Part model, mm, in its own coordinate system. Face numbers are marked on the shaded views. A direction names the side the tool comes from. Round coordinates to 2 decimals unless told otherwise and drop trailing zeros. Loops run counter-clockwise (first coordinate to the right, second up) from the corner with the lowest first, then second, coordinate; pieces in that order, holes last.
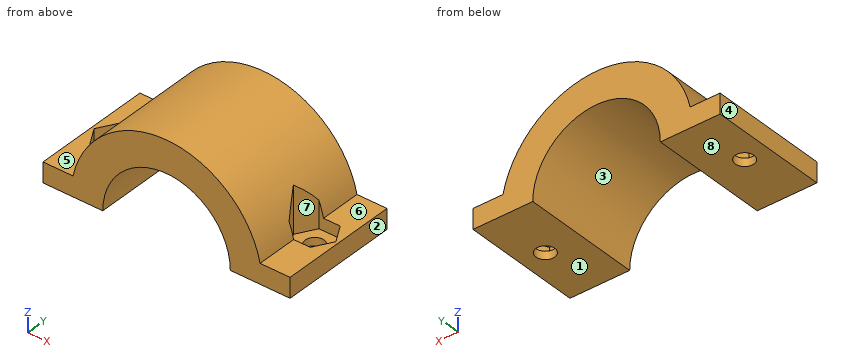
from build123d import *

# Parameters (mm, degrees)
BOSS_EXTRUDE1_DEPTH   = 30
CUT_EXTRUDE1_DEPTH    = 50
SKETCH2_7_R           = 2.35
CUT_EXTRUDE5_DEPTH    = 5
SKETCH2_10_R          = 2.35
CUT_EXTRUDE8_DEPTH    = 3
BODY_MOVE_COPY1_ANGLE = 90


with BuildPart() as part:
    # Sketch1 → Boss-Extrude1 (new body)
    with BuildSketch(Plane(origin=(0, 0, 0), x_dir=(1, 0, 0), z_dir=(0, 1, 0))):
        with BuildLine():
            Line((0, -16), (0, -31))
            Line((0, -31), (-5, -31))
            Line((-5, -31), (-5, -23.473389189))
            ThreePointArc((-5, -23.473389189), (-24, 0), (-5, 23.473389189))
            Line((-5, 23.473389189), (-5, 31))
            Line((-5, 31), (0, 31))
            Line((0, 31), (0, 16))
            ThreePointArc((0, 16), (-16, 0), (0, -16))
        make_face()
    extrude(amount=BOSS_EXTRUDE1_DEPTH)

    # Sketch2 → Cut-Extrude1 (cut)
    with BuildSketch(Plane.ZY.offset(5)):
        Polygon((-23.473389189, 10.375), (-22.329755005, 10.375), (-19.65951001, 15), (-22.329755005, 19.625), (-23.473389189, 19.625), align=None)
        Polygon((23.473389189, 19.625), (22.329755005, 19.625), (19.65951001, 15), (22.329755005, 10.375), (23.473389189, 10.375), align=None)
    extrude(amount=CUT_EXTRUDE1_DEPTH, mode=Mode.SUBTRACT)

    # Sketch2<7> → Cut-Extrude5 (cut)
    with BuildSketch(Plane.ZY.offset(5)):
        with Locations((-25, 15)):
            Circle(SKETCH2_7_R)
        with Locations((25, 15)):
            Circle(SKETCH2_7_R)
    extrude(amount=-CUT_EXTRUDE5_DEPTH, mode=Mode.SUBTRACT)

    # Sketch2<10> → Cut-Extrude8 (cut)
    # profile 1 of 2: a face of its own
    with BuildSketch(Plane.ZY.offset(5)):
        Polygon((-22.329755005, 10.375), (-19.65951001, 15), (-22.329755005, 19.625), (-27.670244995, 19.625), (-30.34048999, 15), (-27.670244995, 10.375), align=None)
        with Locations((-25, 15)):
            Circle(SKETCH2_10_R, mode=Mode.SUBTRACT)
    # profile 2 of 2: a face of its own
    with BuildSketch(Plane.ZY.offset(5)):
        Polygon((27.670244995, 19.625), (30.34048999, 15), (27.670244995, 10.375), (22.329755005, 10.375), (19.65951001, 15), (22.329755005, 19.625), align=None)
        with Locations((25, 15)):
            Circle(SKETCH2_10_R, mode=Mode.SUBTRACT)
    extrude(amount=-CUT_EXTRUDE8_DEPTH, mode=Mode.SUBTRACT)


with BuildPart() as part_1:
    # Body-Move/Copy1: read off the stored shape, not the designer's step
    # Body-Move/Copy1: moved
    add(part.part.moved(Location((0, 0, 16))).rotate(Axis((0, 0, 0), (0, 1, 0)), BODY_MOVE_COPY1_ANGLE))


solid = part_1.part
1) Wall check: line 1 along Y through (x, z) = (-9, 0.8); line 2 along Z through (x, y) = (15.5, 7.25); line 3 along Z through (x, y) = (-11.5, 27.5). Give the ranges that are in metal, low to high.
Values:
line 1: y = 0 to 12.65, 17.35 to 30
line 2: z = 15.99 to 23.99
line 3: z = 0 to 5
2) Slice it at C-C, the plane y = 25.25. Give the cut face in (x, z), then the cut area to 3 significant figures.
Values:
outline: (-15, 0) - (0, 0) arc R16 cw to (32, 0) - (47, 0) - (47, 5) - (39.47, 5) arc R24 ccw to (-7.47, 5) - (-15, 5) - close
area: 574 mm2
3) Drop flat-ended pins along their axis: pin 1 Ø6 at (x, y) = (37, 19.5) entering from +Z; pin 2 Ø4 at (x, y) = (-9, 15) entering from +Z; pin 3 Ø3 at (x, y) = (11, 11.5) entering from -Z; pin 4 Ø3 at (x, y) = (-6.5, 15) entering from +Z. Give the stop position or say it passes through.
Values:
pin 1: stops at z = 15.87
pin 2: passes through
pin 3: stops at z = 14.62
pin 4: stops at z = 2
4) Slice it at D-D, the plane z = 15. Give the cut face in (x, y) (3 decimals).
Values:
outline: (-2.735, 0) - (10.432, 0) - (10.432, 30) - (-2.735, 30) - close; (21.568, 0) - (34.735, 0) - (34.735, 30) - (21.568, 30) - close
5) Slice it at A-A, the plane x = 41. Give the cut face in (y, z) (3 decimals).
Values:
outline: (0, 0) - (12.65, 0) - (12.65, 2) - (10.375, 2) - (10.375, 5) - (0, 5) - close; (17.35, 0) - (30, 0) - (30, 5) - (19.625, 5) - (19.625, 2) - (17.35, 2) - close
6) Mould opens along X. For the marked faces 1, 2, 3 and 4 say: released by +X, released by -X, zero draft, split by the parting line, or undercut.
Values:
face 1: zero draft
face 2: released by +X
face 3: undercut
face 4: released by -X
7) Slice it at B-B, the plane z = 3.5. Give the cut face in (x, y) (1 decimal).
Values:
outline: (-15, 0) - (0.4, 0) - (0.4, 30) - (-15, 30) - close; (31.6, 0) - (47, 0) - (47, 30) - (31.6, 30) - close; hole (-14.3, 15) - (-11.7, 10.4) - (-6.3, 10.4) - (-3.7, 15) - (-6.3, 19.6) - (-11.7, 19.6) - close; hole (35.7, 15) - (38.3, 10.4) - (43.7, 10.4) - (46.3, 15) - (43.7, 19.6) - (38.3, 19.6) - close
8) Tool access for the marked faces 5, 6, 7 and 8: list every direction of +Z, -Z, +X, -X, +Y, -Y with a clear straight run to the whole face (end or side of a thin tool).
Values:
face 5: +Z, -X, +Y, -Y
face 6: +Z, +X, +Y, -Y
face 7: +Z
face 8: -Z, +X, -X, +Y, -Y
